```python
from build123d import *

# Parameters (mm, degrees)
EXTRUDE_1_DEPTH         = 10
HOLE_WIZARD_M36_D       = 3.15
HOLE_WIZARD_M36_DEPTH   = 4
HOLE_WIZARD_M36_TIP     = 0.946355475
HOLE_WIZARD_M36_2_D     = 3.15
HOLE_WIZARD_M36_2_DEPTH = 4
HOLE_WIZARD_M36_2_TIP   = 0.946355475


with BuildPart() as part:
    # Эскиз1 → Бобышка-Вытянуть1 (new body)
    with BuildSketch(Plane(origin=(0, 0, 0), x_dir=(1, 0, 0), z_dir=(0, 1, 0))):
        Polygon((2.886751346, 0), (1.443375673, 2.5), (-1.443375673, 2.5), (-2.886751346, 0), (-1.443375673, -2.5), (1.443375673, -2.5), align=None)
    extrude(amount=EXTRUDE_1_DEPTH)

    # Hole Wizard M36
    with Locations(Plane(origin=(0, 10, 0), x_dir=(1, 0, 0), z_dir=(0, 1, 0))):
        with Locations((0, 0)):
            Hole(HOLE_WIZARD_M36_D / 2, depth=HOLE_WIZARD_M36_DEPTH)
            with Locations((0, 0, -(HOLE_WIZARD_M36_DEPTH + HOLE_WIZARD_M36_TIP / 2))):  # 118° drill point
                Cone(0, HOLE_WIZARD_M36_D / 2, HOLE_WIZARD_M36_TIP, mode=Mode.SUBTRACT)

    # Hole Wizard M36 2
    with Locations(Plane(origin=(0, 0, 0), x_dir=(-1, 0, 0), z_dir=(0, -1, 0))):
        with Locations((0, 0)):
            Hole(HOLE_WIZARD_M36_2_D / 2, depth=HOLE_WIZARD_M36_2_DEPTH)
            with Locations((0, 0, -(HOLE_WIZARD_M36_2_DEPTH + HOLE_WIZARD_M36_2_TIP / 2))):  # 118° drill point
                Cone(0, HOLE_WIZARD_M36_2_D / 2, HOLE_WIZARD_M36_2_TIP, mode=Mode.SUBTRACT)


solid = part.part
```
Model file for the job. Use its own axes, mm. A direction names the side the tool comes from. Give positions to 0.01 mm unless a question says otherwise; leave off trailing zeros. Write each loop counter-clockwise with the first axis right and the second up, starting at its lowest first coordinate (ties: lowest second). Pieces come first, ordered by that corner, then holes. Notation, with made-up numbers: (67.25, 16) -> (77.25, 16) arc R19 cw to (77.25, 42) -> close; hole circle Ø9 at (42.25, 10). An arc over 180 degrees is marked (long way). Use CSV: the item, a comma, the result in double quotes. Start each with the question number.
1) Cut at C-C on z = -1.85. List the corners of the cut face in (x, y).
2) Cut at A-A on y = 3.5. List the corners of the cut face in (x, z) (3 decimals).
3) Drill centre lines: L1, parallel to Z at x = 0, y = 1.95 (3 decimals); L2, parallel to X at y = 5.5, z = 0.3; L3, parallel to X at y = 5.75, z = -0.35. Where is each one in solid material? Low to high.
4) Pin check, flat tip, straight feed: P1, Ø1.5, axis at x = 0.5, z = 0.5, coming from the +Y side. Stop position of the tip, or through.
5) Tool access for faces 5 (the cylindrical face through (-1.25, 2.03, 0.96)), 6 (the cylindrical face through (1.25, 7.97, 0.96)), 7 (the flat face through (0, 5, -2.5)): list every direction of +Z, -Z, +X, -X, +Y, -Y with a clear straight run to the whole face (end or side of a thin tool).
6) Cut at B-B on y = 5.75. List the corners of the cut face in (x, z).
7) Two-plate mould, pull along Z, no slides. Class faces 1 (the flat face through (2.155, 4.93, 1.267)), 2 (the flat face through (-2.155, 4.93, -1.267)), 3 (the conical face through (-0.261, 4.782, -0.082)), 4 (the flat face through (0, 10, -2)): released by +Z, released by -Z, zero draft, split by the parting line, or undercut.
8) Cut at D-D on x = 1.7. List the corners of the cut face in (y, z).
Final values:
1,outline,"(-1.82, 0) -> (1.82, 0) -> (1.82, 10) -> (-1.82, 10) -> close"
2,outline,"(-2.887, 0) -> (-1.443, -2.5) -> (1.443, -2.5) -> (2.887, 0) -> (1.443, 2.5) -> (-1.443, 2.5) -> close; hole circle Ø3.15 at (0, 0)"
3,L1,"z = -2.5 to -1.575, 1.575 to 2.5"
3,L2,"x = -2.71 to -0.68, 0.68 to 2.71"
3,L3,"x = -2.68 to -1.1, 1.1 to 2.68"
4,P1,"stops at y = 5.93"
5,face 5,"-Y"
5,face 6,"+Y"
5,face 7,"-Z, +X, -X, +Y, -Y"
6,outline,"(-2.89, 0) -> (-1.44, -2.5) -> (1.44, -2.5) -> (2.89, 0) -> (1.44, 2.5) -> (-1.44, 2.5) -> close; hole circle Ø2.32 at (0, 0)"
7,face 1,"released by +Z"
7,face 2,"released by -Z"
7,face 3,"undercut"
7,face 4,"zero draft"
8,outline,"(0, -2.06) -> (10, -2.06) -> (10, 2.06) -> (0, 2.06) -> close"
